Part model, mm, in its own coordinate system. A direction names the side the tool comes from. Coordinates: 2 decimals unless noted, no trailing zeros. Write each loop counter-clockwise with the first axis right and the second up, starting at its lowest first coordinate (ties: lowest second). Pieces come first, ordered by that corner, then holes. Notation, with made-up numbers: (77.5, -4) -> (135.5, -4) arc R20 cw to (135.5, 29) -> close; hole circle Ø9 at (49.5, 76.5). An arc over 180 degrees is marked (long way). One line per question, with ' | ' between items. Start each with the question number.
Item 1: Saw through at C-C (x = 65). List the corners of the cut face in (y, z), and give its area (3 significant figures).
Item 2: Probe probe 1 along X at (y, z) = (-49.5, 12); probe 2 along Z at (x, y) = (64, -84.5); probe 3 along Y at (x, z) = (68, 14). List the from-to ranges inside material, lowest first. Write a range as [from, to].
Item 3: Saw through at D-D (z = 56). List the corners of the cut face in (x, y).
Item 4: Two-plate mould, pull along Y, no slides. Class faces 5 (the flat face through (100.219, -28.737, 4.93)), 6 (the cylindrical face through (72.153, -9.86, 71.103)), 7 (the flat face through (66, 0, 70)): pulls with the +Y half, pulls with the -Y half, needs draft (parallel to the pull), parting line crosses it, or undercut.
Item 5: Saw through at B-B (y = -17). List the corners of the cut face in (x, z) (3 decimals).
Item 6: Saw through at A-A (z = 12). List the corners of the cut face in (x, y), and give its area (3 significant figures).
Item 7: Pin check, flat tips, straight feed: pin 1 (6 mm diameter, centred on x = 79.5, z = 67, fed in from -Y); pin 2 (7.5 mm diameter, centred on x = 103.5, y = -17, fed in from +Z); pin 3 (4 mm diameter, centred on y = -93.5, z = 36, fed in from +X). Stop position of each tip, or through.
Item 8: 3-axis set-ups, long thin cutter, end or side, ignore diameter. For faces 1 (the flat face through (27.006, -100.787, 9.86)), 2 (the cylindrical face through (9.86, -75.31, 76.43)), 3 (the flat face through (100.787, -9.86, 27.006)), 4 (the flat face through (70.44, -76.87, 14.93)): which of +Z, -Z, +X, -X, +Y, -Y reach the whole face in a straight line?
from build123d import *

# Parameters (mm, degrees)
F1_ANGLE  = 90
F3_DEPTH  = 20
F5_DEPTH  = 20
F7_DEPTH  = 20
F10_DEPTH = 10


with BuildPart() as f1:
    # F0 (on Right) → F1 (revolve)
    with BuildSketch(Plane.YZ):
        with BuildLine():
            Line((0, 94.3), (0, 114.3))
            ThreePointArc((0, 114.3), (-80.8223050896, 80.8223050896), (-114.3, 0))
            Line((-114.3, 0), (-94.3, 0))
            ThreePointArc((-94.3, 0), (-66.6801694659, 66.6801694659), (0, 94.3))
        make_face()
    revolve(axis=Axis((0, 0, 104.3), (0, 0, 1)), revolution_arc=F1_ANGLE)

    # F2 (on face) → F3 (cut)
    with BuildSketch(Plane(origin=(0, 0, 0), x_dir=(-1, 0, 0), z_dir=(0, 1, 0))):
        with BuildLine():
            Line((-26.2183692689, 97.8482862031), (-27.7712835395, 103.6438411608))
            ThreePointArc((-27.7712835395, 103.6438411608), (-75.8725576213, 75.8725576213), (-103.6438411608, 27.7712835395))
            Line((-103.6438411608, 27.7712835395), (-97.8482862031, 26.2183692689))
            ThreePointArc((-97.8482862031, 26.2183692689), (-71.6299169342, 71.6299169342), (-26.2183692689, 97.8482862031))
        make_face()
    extrude(amount=-F3_DEPTH, mode=Mode.SUBTRACT)

    # F4 (on face) → F5 (cut)
    with BuildSketch(Plane.YZ):
        with BuildLine():
            ThreePointArc((-97.8482862031, 26.2183692689), (-71.6299169342, 71.6299169342), (-26.2183692689, 97.8482862031))
            Line((-26.2183692689, 97.8482862031), (-27.7712835395, 103.6438411608))
            ThreePointArc((-27.7712835395, 103.6438411608), (-75.8725576213, 75.8725576213), (-103.6438411608, 27.7712835395))
            Line((-103.6438411608, 27.7712835395), (-97.8482862031, 26.2183692689))
        make_face()
    extrude(amount=F5_DEPTH, mode=Mode.SUBTRACT)

    # F6 (on face) → F7 (cut)
    with BuildSketch(Plane(origin=(0, 0, 0), x_dir=(1, 0, 0), z_dir=(0, 0, -1))):
        with BuildLine():
            Line((27.7712835395, 103.6438411608), (26.2183692689, 97.8482862031))
            ThreePointArc((26.2183692689, 97.8482862031), (40.3932806821, 92.8981855352), (53.6808214668, 85.9072721406))
            Line((53.6808214668, 85.9072721406), (56.8603370522, 90.9955607176))
            ThreePointArc((56.8603370522, 90.9955607176), (42.7857750957, 98.4005459815), (27.7712835395, 103.6438411608))
        make_face()
        with BuildLine():
            ThreePointArc((84.9573285329, 55.171934247), (92.1790767398, 42.0084254811), (97.3758097986, 27.9220641443))
            Line((97.3758097986, 27.9220641443), (103.1433799742, 29.5758882792))
            ThreePointArc((103.1433799742, 29.5758882792), (97.6388443651, 44.496584937), (89.9893519405, 58.4397684571))
            Line((89.9893519405, 58.4397684571), (84.9573285329, 55.171934247))
        make_face()
    extrude(amount=-F7_DEPTH, mode=Mode.SUBTRACT)

    # F9 (on offset) → F10 (cut)
    with BuildSketch(Plane(origin=(0, 0, 10), x_dir=(1, 0, 0), z_dir=(0, 0, -1))):
        with BuildLine():
            ThreePointArc((97.3758097986, 27.9220641443), (99.4762319066, 19.1355503099), (100.7854867979, 10.1968451452))
            Line((100.7854867979, 10.1968451452), (106.7579299629, 10.7719260129))
            ThreePointArc((106.7579299629, 10.7719260129), (105.3709505868, 20.2546975401), (103.1433799742, 29.5758882792))
            Line((103.1433799742, 29.5758882792), (97.3758097986, 27.9220641443))
        make_face()
        Polygon((0.327321584, 0.5238240331), (0, 0), (0.4947707785, 0.5399475566), align=None)
        Polygon((0.4947707785, 0.5399475566), (0, 0), (2.5848787999, 0.7412020686), align=None)
        with BuildLine():
            Line((56.8603370522, 90.9955607176), (53.6808214668, 85.9072721406))
            ThreePointArc((53.6808214668, 85.9072721406), (61.3162809887, 80.6350028568), (68.4372880315, 74.6861942189))
            Line((68.4372880315, 74.6861942189), (72.4908292772, 79.1098582397))
            ThreePointArc((72.4908292772, 79.1098582397), (64.948044917, 85.411014872), (56.8603370522, 90.9955607176))
        make_face()
    extrude(amount=-F10_DEPTH, mode=Mode.SUBTRACT)


solid = f1.part
From the geometry:
1) outline: (-94.02, 0) -> (-68.32, 0) arc R68.32 cw to (0, 68.32) -> (0, 77.7) -> (-20, 77.7) -> (-20, 85.37) -> (0, 85.37) -> (0, 94.02) arc R94.02 ccw to start; hole (-85.37, 10) -> (-77.7, 10) -> (-77.7, 20) -> (-85.37, 20) -> close | area: 3,050 mm2
2) probe 1: [79.36, 88.38], [95.2, 102.32] | probe 2: [0, 10], [20, 42.76] | probe 3: [-90.8, -83], [-75.08, -63.82]
3) outline: (0, -99.64) arc R99.64 ccw to (99.64, 0) -> (91.53, 0) -> (91.53, -20) -> (84.41, -20) -> (84.41, 0) -> (75.87, 0) arc R75.87 cw to (0, -75.87) -> (0, -84.41) -> (20, -84.41) -> (20, -91.53) -> (0, -91.53) -> close
4) face 5: undercut | face 6: needs draft | face 7: pulls with the +Y half
5) outline: (0, 92.755) arc R92.755 cw to (92.755, 0) -> (113.029, 0) arc R113.029 ccw to (0, 113.029) -> close; hole (26.218, 97.848) arc R101.3 cw to (97.848, 26.218) -> (103.644, 27.771) arc R107.3 ccw to (27.771, 103.644) -> close; hole (99.863, 10) -> (105.945, 10) -> (105.945, 20) -> (99.863, 20) -> close
6) outline: (0, -113.67) arc R113.67 ccw to (113.67, 0) -> (93.53, 0) arc R93.53 cw to (0, -93.53) -> close; hole (26.22, -97.85) -> (27.77, -103.64) arc R107.3 ccw to (72.49, -79.11) -> (68.44, -74.69) arc R101.3 cw to start; hole (84.96, -55.17) -> (89.99, -58.44) arc R107.3 ccw to (106.76, -10.77) -> (100.79, -10.2) arc R101.3 cw to start | area: 2,680 mm2
7) pin 1: y = -53.57 | pin 2: z = 53.25 | pin 3: x = 58.51
8) face 1: -Z | face 2: -X | face 3: +Y | face 4: none
